Check sheet for the modelled part. Datum: model origin and axes. Units: mm. Face numbers are marked on the shaded views. A direction names the side the tool comes from. Round coordinates to 2 decimals unless told otherwise and drop trailing zeros. Write each loop counter-clockwise with the first axis right and the second up, starting at its lowest first coordinate (ties: lowest second). Pieces come first, ordered by that corner, then holes. Notation, with made-up numbers: (70, 85) -> (121, 85) arc R12 cw to (121, 96) -> close; hole circle Ø9 at (70, 48.25). An arc over 180 degrees is marked (long way). One line per item, written item: value. Start each with the question number.
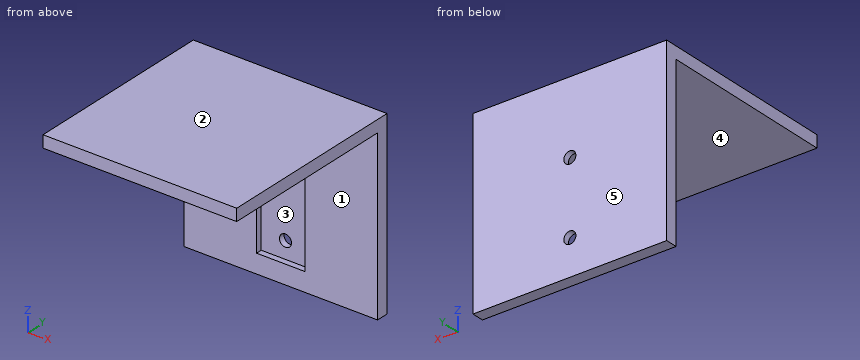
```python
from build123d import *

# Parameters (mm, degrees)
F0_W     = 75
F0_H     = 5
F1_DEPTH = 80
F2_W     = 20
F2_H     = 50
F3_DEPTH = 2.5
F5_D     = 5


with BuildPart() as f1:
    # F0 (on Right) → F1 (new body)
    with BuildSketch(Plane.YZ):
        with Locations((-37.5, 2.5)):
            Rectangle(F0_W, F0_H)
        Polygon((5, 5), (0, 5), (0, 0), (0, -70), (5, -70), align=None)
    extrude(amount=F1_DEPTH)

    # F2 (on Front) → F3 (cut)
    with BuildSketch(Plane.XZ):
        with Locations((39.995763, -37.202657)):
            Rectangle(F2_W, F2_H)
    extrude(amount=-F3_DEPTH, mode=Mode.SUBTRACT)

    # F5 (through all)
    with Locations(Plane.XZ):
        with Locations((40.000014, -25.175888), (40.000014, -55.175888)):
            Hole(F5_D / 2)


solid = f1.part
```
1. Depth check by flat-ended pin: pin 1 Ø22.5 at (x, y) = (46.5, -43.5) entering from -Z; pin 2 Ø1 at (x, z) = (9, -27) entering from -Y; pin 3 Ø6 at (x, z) = (37, -26.5) entering from -Y; pin 4 Ø6 at (x, z) = (40, -55.18) entering from +Y. Enter the tip coordinate at first touch or a pass-through.
2. Release check for a two-part mould opening along Z. For the marked faces 1, 2 and 3 record: +Z half, -Z half, draft (parallel to the pull), parting line (faces both ways), or undercut.
3. Cross-section at B-B (z = -30.5). Record the cut outline in (x, y).
4. Cross-section at D-D (x = 16.5). Record the cut outline in (y, z), plus the area to 3 significant figures.
5. Material ranges on probe 1 along Y at (x, z) = (20.5, -45.5); probe 2 along Y at (x, z) = (49, -45), recorded low to high.
6. Cross-section at C-C (y = -20). Record the cut outline in (x, z), plus the area to 3 significant figures.
7. Cross-section at A-A (x = 40). Record the cut outline in (y, z), plus the area to 3 significant figures.
8. Access from +Z, -Z, +X, -X, +Y, -Y to the whole of each face (thin tool, end or side, straight path). Record for the marked faces 4 and 5.
Working result:
1. pin 1: stops at z = 0
1. pin 2: stops at y = 0
1. pin 3: stops at y = 2.5
1. pin 4: stops at y = 5
2. face 1: draft
2. face 2: +Z half
2. face 3: undercut
3. outline: (0, 0) -> (30, 0) -> (30, 2.5) -> (50, 2.5) -> (50, 0) -> (80, 0) -> (80, 5) -> (0, 5) -> close
4. outline: (-75, 0) -> (0, 0) -> (0, -70) -> (5, -70) -> (5, 5) -> (-75, 5) -> close
4. area: 750 mm^2
5. probe 1: y = 0 to 5
5. probe 2: y = 2.5 to 5
6. outline: (0, 0) -> (80, 0) -> (80, 5) -> (0, 5) -> close
6. area: 400 mm^2
7. outline: (-75, 0) -> (0, 0) -> (0, -12.2) -> (2.5, -12.2) -> (2.5, -22.68) -> (5, -22.68) -> (5, 5) -> (-75, 5) -> close; (0, -70) -> (5, -70) -> (5, -57.68) -> (2.5, -57.68) -> (2.5, -62.2) -> (0, -62.2) -> close; (2.5, -52.68) -> (5, -52.68) -> (5, -27.68) -> (2.5, -27.68) -> close
7. area: 600 mm^2
8. face 4: -Z, +X, -X, -Y
8. face 5: +Z, -Z, +X, -X, +Y
